Autodesk Inventor part; units mm, degrees
ref_plane "ANBAU_XY" through (0, 0, 0) normal (0, 0, 1) x (1, 0, 0)
ref_plane "ANBAU_YZ" through (0, 0, 0) normal (1, 0, 0) x (0, 1, 0)
ref_plane "ANBAU_ZX" through (0, 0, 0) normal (0, 1, 0) x (0, 0, 1)
sketch "Sketch_1" plane through (0, 0, 0) normal (1, 0, 0) x (0, 1, 0)
  line L0 (0, -78.5) -> (0, 0)
  line L1 (0, 0) -> (14, 0)
  line L2 (14, 0) -> (14, -47.58)
  line L3 (14, -47.58) -> (13.08, -48.5)
  line L4 (13.08, -48.5) -> (12, -48.5)
  line L5 (12, -48.5) -> (12, -78)
  line L6 (12, -78) -> (11.5, -78.5)
  line L7 (11.5, -78.5) -> (0, -78.5)
  line L8 (0, -78.5) -> (0, 0)
revolve "Revolution1" add sketch "Sketch_1" angle 360 about axis through (0, 0, -78.5) along (0, 0, -1)
thread "Thread1"
ref_plane "ANBAU_XY" through (0, 0, 0) normal (0, 0, 1) x (1, 0, 0)
ref_plane "ANBAU_YZ" through (0, 0, 0) normal (1, 0, 0) x (0, 1, 0)
ref_plane "ANBAU_ZX" through (0, 0, 0) normal (0, 1, 0) x (0, 0, 1)
properties part number "ESBF-BS-100-ESBF-BS-100---(KSA)"
The model under review builds one solid part; all positions refer to its coordinate system, in mm. A direction names the side the tool comes from. Coordinates: 2 decimals unless noted, no trailing zeros. Loops run counter-clockwise (first coordinate to the right, second up) from the corner with the lowest first, then second, coordinate; pieces in that order, holes last.
(1) Consider section D-D, the plane z = -55. Give the boundary of the cut face in (x, y), plus the area to 3 significant figures.
Determined:
outline: circle Ø24 at (0, 0)
area: 452 mm2
(2) Consider section C-C, the plane z = -9.5. Give the boundary of the cut face in (x, y), plus the area to 3 significant figures.
Determined:
outline: circle Ø28 at (0, 0)
area: 616 mm2
(3) Consider section A-A, the plane x = 0. Give the boundary of the cut face in (y, z), plus the area to 3 significant figures.
Determined:
outline: (-14, -47.58) - (-13.08, -48.5) - (-12, -48.5) - (-12, -78) - (-11.5, -78.5) - (11.5, -78.5) - (12, -78) - (12, -48.5) - (13.08, -48.5) - (14, -47.58) - (14, 0) - (-14, 0) - close
area: 2,080 mm2
(4) Insertion check: P1, Ø4, axis at y = 7, z = -27.5, coming from the -X side; P2, Ø3, axis at x = -8, z = -16.5, coming from the -Y side; P3, Ø10, axis at y = 4, z = -12.5, coming from the -X side; P4, Ø4, axis at x = -0.5, z = -59.5, coming from the -Y side. Each pin has a flat end and moves straight along its axis. Give the tip position at first contact, or say it passes through.
Determined:
P1: stops at x = -13.08
P2: stops at y = -12.4
P3: stops at x = -14
P4: stops at y = -12
(5) Tool access review of faces 1 (the cylindrical face through (-5.362, 12.932, -24.123)), 2 (the flat face through (-11, 6, -48.5)): name each direction out of +Z, -Z, +X, -X, +Y, -Y from which nothing blocks a thin tool from reaching the whole face with its end or side.
Determined:
face 1: +Z, -Z
face 2: -Z
(6) Wall thickness on L1, parallel to Z at x = -7.5, y = -9.5; L2, parallel to Y at x = -5, z = -39.5: over which ranges is each line inside the solid? List them lowest first.
Determined:
L1: z = -48.5 to 0
L2: y = -13.08 to 13.08
